Check sheet for the modelled part. Datum: model origin and axes. Units: mm. A direction names the side the tool comes from. Round coordinates to 2 decimals unless told otherwise and drop trailing zeros. Order: outer loops, then holes, each group sorted by start corner. A loop starts at its lowest first (then second) coordinate and runs counter-clockwise, first axis right, second up.
(1) Mould release check, pull along Z, two halves, no side actions. Record for faces 1 (the flat face through (-23.02, -9.69, 5.46)), 2 (the cylindrical face through (0.28, 17.87, -26.77)), 3 (the flat face through (25, 3, -30)), 4 (the cylindrical face through (-0.448, -0.541, 0.887)): released by +Z, released by -Z, zero draft, split by the parting line, or undercut.
(2) Sectioned sample at A-A, the plane y = 11.5. Enter the section's corners in (x, z).
(3) Sectioned sample at C-C, the plane z = -28.6. Enter the section's corners in (x, y).
(4) Sectioned sample at D-D, the plane z = -13.5. Enter the section's corners in (x, y).
(5) Depth check by flat-ended pin: pin 1 (3.5 mm diameter, centred on x = 2, y = -9.5, fed in from +Z); pin 2 (1.5 mm diameter, centred on x = 7.5, z = -27.5, fed in from -Y); pin 3 (2 mm diameter, centred on x = -25.5, y = -12.5, fed in from -Z); pin 4 (3 mm diameter, centred on x = -8, z = -21, fed in from +Y). Enter the tip coordinate at first touch or a pass-through.
(6) Tool access check on faces 5 (the flat face through (3, -11, 4.4)), 6 (the flat face through (0, 2.4, -9)), 7 (the flat face through (0, 5, 0)). Record the directions out of +Z, -Z, +X, -X, +Y, -Y that give a thin tool (end or side, any length) a straight path to the whole face; none if there is none.
(7) Thickness scan on probe 1 along Z at (x, y) = (22, 3.4); probe 2 along Z at (x, y) = (-22, 0.95); probe 3 along Y at (x, z) = (-26.5, 9). Record the ranges inside material, lowest first.
```python
from build123d import *

# Parameters (mm, degrees)
PAD001_DEPTH                  = 32
SKETCH010_R                   = 20.25
SKETCH010_R_2                 = 7.8
POCKET_DEPTH                  = 2.6
SKETCH011_R                   = 2.75
POCKET001_DEPTH               = 23.001
SKETCH014_R                   = 5.5
POCKET004_DEPTH               = 2
SKETCH008_R                   = 5
PAD002_DEPTH                  = 17.8
SKETCH012_R                   = 1.3
POCKET002_DEPTH               = 10
SKETCH013_R                   = 2.75
POCKET003_DEPTH               = 18.001
SKETCH015_R                   = 5.5
POCKET005_DEPTH               = 2
CHAMFER_SIZE                  = 2
CHAMFER001_SIZE               = 1.85
CHAMFER002_SIZE               = 0.5
FILLET_R                      = 4.4
BODY001082169_ROLL_ANGLE      = 90
BODY001082169_PLACEMENT_ANGLE = 180


with BuildPart() as part:
    # Sketch009 → Pad001 (new body, symmetric)
    with BuildSketch(Plane.YZ):
        with BuildLine():
            Line((-36.6, 0), (-36.6, 5))
            Line((-36.6, 5), (18, 5))
            Line((18, 5), (18, 0))
            Line((18, 0), (8.4, 0))
            ThreePointArc((8.4, 0), (6.985786, -0.585786), (6.4, -2))
            Line((6.4, -2), (6.4, -18))
            Line((6.4, -18), (1.4, -18))
            Line((1.4, -18), (1.4, -1.8))
            ThreePointArc((1.4, -1.8), (0.872792, -0.527208), (-0.4, 0))
            Line((-0.4, 0), (-36.6, 0))
        make_face()
    extrude(amount=PAD001_DEPTH, both=True)

    # Sketch010 → Pocket (cut)
    with BuildSketch(Plane.XY.offset(5)):
        Circle(SKETCH010_R)
        Circle(SKETCH010_R_2, mode=Mode.SUBTRACT)
    extrude(amount=-POCKET_DEPTH, mode=Mode.SUBTRACT)

    # Sketch011 → Pocket001 (cut, through all)
    with BuildSketch(Plane.XY.offset(5)):
        with Locations((22, -28.6)):
            Circle(SKETCH011_R)
        with Locations((-22, -28.6)):
            Circle(SKETCH011_R)
        with BuildLine():
            ThreePointArc((-26.457513, 18), (-30.583005, 9.416995), (-32, 0))
            Line((-32, 0), (-33, 0))
            Line((-33, 0), (-33, 19))
            Line((-33, 19), (33, 19))
            Line((33, 19), (33, 0))
            Line((33, 0), (32, 0))
            ThreePointArc((32, 0), (30.583005, 9.416995), (26.457513, 18))
            Line((-26.457513, 18), (26.457513, 18))
        make_face()
    extrude(amount=-POCKET001_DEPTH, mode=Mode.SUBTRACT)

    # Sketch014 → Pocket004 (cut)
    with BuildSketch(Plane.XY.offset(5)):
        with Locations((-22, -28.6)):
            Circle(SKETCH014_R)
        with Locations((22, -28.6)):
            Circle(SKETCH014_R)
    extrude(amount=-POCKET004_DEPTH, mode=Mode.SUBTRACT)

    # Sketch008 → Pad002 (join)
    with BuildSketch(Plane.XY.offset(5)):
        with Locations((-22.083648, 12.75)):
            Circle(SKETCH008_R)
        with Locations((22.083648, 12.75)):
            Circle(SKETCH008_R)
        with Locations((0, -25.5)):
            Circle(SKETCH008_R)
    extrude(amount=PAD002_DEPTH)

    # Sketch012 → Pocket002 (cut)
    with BuildSketch(Plane.XY.offset(22.8)):
        with Locations((-22.083648, 12.75)):
            Circle(SKETCH012_R)
        with Locations((22.083648, 12.75)):
            Circle(SKETCH012_R)
        with Locations((0, -25.5)):
            Circle(SKETCH012_R)
    extrude(amount=-POCKET002_DEPTH, mode=Mode.SUBTRACT)

    # Sketch013 → Pocket003 (cut, through all)
    with BuildSketch(Plane.XZ):
        with Locations((0, -10)):
            Circle(SKETCH013_R)
        Polygon((-32, -2), (-16, -18), (16, -18), (32, -2), (33, -2), (33, -20), (-33, -20), (-33, -2), align=None)
    extrude(amount=-POCKET003_DEPTH, mode=Mode.SUBTRACT)

    # Sketch015 → Pocket005 (cut)
    with BuildSketch(Plane(origin=(0, 6.4, 0), x_dir=(0.999848, 0, 0.017452), z_dir=(0, -1, 0))):
        with Locations((-0.174524, -9.998477)):
            Circle(SKETCH015_R)
    extrude(amount=POCKET005_DEPTH, mode=Mode.SUBTRACT)

    # Chamfer
    chamfer_edges = [part.edges().sort_by_distance(p)[0] for p in [
        (29.066737, 13.383751, 0),
        (31.225598, 6.997288, -0.574378),
        (-29.066737, 13.383751, 0),
        (-31.225598, 6.997288, -0.574378),
    ]]
    chamfer(chamfer_edges, length=CHAMFER_SIZE)

    # Chamfer001
    chamfer001_edges = [part.edges().sort_by_distance(p)[0] for p in [
        (22.676734, 6.4, -11.323266),
        (0, 6.4, -18),
        (-22.676734, 6.4, -11.323266),
        (-32, -36.6, 2.5),
        (32, -36.6, 2.5),
    ]]
    chamfer(chamfer001_edges, length=CHAMFER001_SIZE)

    # Chamfer002
    chamfer002_edges = [part.edges().sort_by_distance(p)[0] for p in [
        (-27.5, -28.6, 5),
        (16.5, -28.6, 5),
        (-7.8, 0, 5),
        (-5.499162, 6.4, -10.095988),
    ]]
    chamfer(chamfer002_edges, length=CHAMFER002_SIZE)

    # Fillet
    fillet_edges = [part.edges().sort_by_distance(p)[0] for p in [
        (-26.457513, 18, 3.5),
        (26.457513, 18, 3.5),
    ]]
    fillet(fillet_edges, radius=FILLET_R)


with BuildPart() as part_1:
    # Body001082169 roll: moved
    add(part.part.rotate(Axis((0, 0, 0), (1, 0, 0)), BODY001082169_ROLL_ANGLE))


with BuildPart() as part_2:
    # Body001082169 placement: moved
    add(part_1.part.rotate(Axis((0, 0, 0), (0, 0, 1)), BODY001082169_PLACEMENT_ANGLE))


solid = part_2.part
```
Derived:
1. face 1: released by +Z
1. face 2: undercut
1. face 3: undercut
1. face 4: released by -Z
2. outline: circle Ø10 at (-22.08, 12.75); circle Ø10 at (0, -25.5); circle Ø10 at (22.08, 12.75)
3. outline: (-32, 0) - (-24.75, 0) - (-24.75, 3) - (-27.5, 3) - (-27.5, 4.5) - (-28, 5) - (-32, 5) - close; (-19.25, 0) - (19.25, 0) - (19.25, 3) - (16.5, 3) - (16.5, 4.5) - (16, 5) - (3.92, 5) - (3.92, 22.8) - (-3.92, 22.8) - (-3.92, 5) - (-16, 5) - (-16.5, 4.5) - (-16.5, 3) - (-19.25, 3) - close; (24.75, 0) - (32, 0) - (32, 5) - (28, 5) - (27.5, 4.5) - (27.5, 3) - (24.75, 3) - close
4. outline: (-32, 0) - (32, 0) - (32, 5) - (15.09, 5) - (15.09, 2.4) - (-15.09, 2.4) - (-15.09, 5) - (-32, 5) - close
5. pin 1: stops at z = 4.4
5. pin 2: stops at y = 0
5. pin 3: passes through
5. pin 4: stops at y = 5
6. face 5: +Z
6. face 6: +Y
6. face 7: +Z, +X, -X, +Y
7. probe 1: z = -36.6 to -34.1, -23.1 to 18
7. probe 2: z = -36.6 to -31.35, -25.85 to 18
7. probe 3: y = 0 to 5
